from build123d import *

# Parameters (mm, degrees)
F0_W     = 1.2
F0_H     = 7
F1_DEPTH = 1.3
F2_DEPTH = 4.9
F3_DEPTH = 4


with BuildPart() as f1:
    # F0 (on Top) → F1 (new body)
    with BuildSketch(Plane.XY):
        with BuildLine():
            Line((9.05, 3.5), (6.914658, 3.5))
            ThreePointArc((6.914658, 3.5), (-4.806972, 6.079105), (-5, -5.92136))
            ThreePointArc((-5, -5.92136), (0, -7.75), (5, -5.92136))
            ThreePointArc((5, -5.92136), (6.079105, -4.806972), (6.914658, -3.5))
            Line((6.914658, -3.5), (9.05, -3.5))
            Line((9.05, -3.5), (9.05, 3.5))
        make_face()
        with BuildLine():
            ThreePointArc((-5, -5.92136), (-4.806972, 6.079105), (6.914658, 3.5))
            Line((6.914658, 3.5), (9.05, 3.5))
            Line((9.05, 3.5), (10.25, 3.5))
            Line((10.25, 3.5), (10.25, 4.5))
            Line((10.25, 4.5), (7.966963, 4.5))
            ThreePointArc((7.966963, 4.5), (-6.259851, 6.673588), (-5, -7.663061))
            Line((-5, -7.663061), (-5, -5.92136))
        make_face()
        with BuildLine():
            ThreePointArc((5, -5.92136), (0, -7.75), (-5, -5.92136))
            Line((-5, -5.92136), (-5, -7.663061))
            ThreePointArc((-5, -7.663061), (0, -9.15), (5, -7.663061))
            Line((5, -7.663061), (5, -5.92136))
        make_face()
        with Locations((9.65, 0)):
            Rectangle(F0_W, F0_H)
        with BuildLine():
            ThreePointArc((6.914658, -3.5), (6.079105, -4.806972), (5, -5.92136))
            Line((5, -5.92136), (5, -7.663061))
            ThreePointArc((5, -7.663061), (6.673588, -6.259851), (7.966963, -4.5))
            Line((7.966963, -4.5), (10.25, -4.5))
            Line((10.25, -4.5), (10.25, -3.5))
            Line((10.25, -3.5), (9.05, -3.5))
            Line((9.05, -3.5), (6.914658, -3.5))
        make_face()
    extrude(amount=F1_DEPTH)

    # F0 (on Top) → F2 (join)
    with BuildSketch(Plane.XY):
        with BuildLine():
            ThreePointArc((-5, -5.92136), (-4.806972, 6.079105), (6.914658, 3.5))
            Line((6.914658, 3.5), (9.05, 3.5))
            Line((9.05, 3.5), (10.25, 3.5))
            Line((10.25, 3.5), (10.25, 4.5))
            Line((10.25, 4.5), (7.966963, 4.5))
            ThreePointArc((7.966963, 4.5), (-6.259851, 6.673588), (-5, -7.663061))
            Line((-5, -7.663061), (-5, -5.92136))
        make_face()
        with BuildLine():
            ThreePointArc((6.914658, -3.5), (6.079105, -4.806972), (5, -5.92136))
            Line((5, -5.92136), (5, -7.663061))
            ThreePointArc((5, -7.663061), (6.673588, -6.259851), (7.966963, -4.5))
            Line((7.966963, -4.5), (10.25, -4.5))
            Line((10.25, -4.5), (10.25, -3.5))
            Line((10.25, -3.5), (9.05, -3.5))
            Line((9.05, -3.5), (6.914658, -3.5))
        make_face()
    extrude(amount=F2_DEPTH)

    # F0 (on Top) → F3 (join)
    with BuildSketch(Plane.XY):
        with Locations((9.65, 0)):
            Rectangle(F0_W, F0_H)
    extrude(amount=F3_DEPTH)


solid = f1.part
Model file for the job. Use its own axes, mm. A direction names the side the tool comes from. Give positions to 0.01 mm unless a question says otherwise; leave off trailing zeros. Write each loop counter-clockwise with the first axis right and the second up, starting at its lowest first coordinate (ties: lowest second). Pieces come first, ordered by that corner, then holes. Notation, with made-up numbers: (1.5, 62) -> (45.5, 62) arc R27 cw to (45.5, 99) -> close; hole circle Ø10 at (-20.75, -19.75). An arc over 180 degrees is marked (long way). Write item = value, one per line.
(1) Slice it at B-B, the plane z = 2.4. Give the cut face in (x, y).
Determined:
outline = (-5, -7.66) -> (-5, -5.92) arc R7.75 cw (long way) to (6.91, 3.5) -> (9.05, 3.5) -> (9.05, -3.5) -> (6.91, -3.5) arc R7.75 cw to (5, -5.92) -> (5, -7.66) arc R9.15 ccw to (7.97, -4.5) -> (10.25, -4.5) -> (10.25, 4.5) -> (7.97, 4.5) arc R9.15 ccw (long way) to start
(2) Slice it at C-C, the plane y = 0. Give the cut face in (x, z).
Determined:
outline = (-9.15, 0) -> (10.25, 0) -> (10.25, 4) -> (9.05, 4) -> (9.05, 1.3) -> (-7.75, 1.3) -> (-7.75, 4.9) -> (-9.15, 4.9) -> close
(3) Slice it at A-A, the plane x = 8.25. Give the cut face in (y, z), then the cut area to 3 significant figures.
Determined:
outline = (-4.5, 0) -> (4.5, 0) -> (4.5, 4.9) -> (3.5, 4.9) -> (3.5, 1.3) -> (-3.5, 1.3) -> (-3.5, 4.9) -> (-4.5, 4.9) -> close
area = 18.9 mm2
(4) Tool access for faces 1 (the face through (9, 4.5, 2)), 2 (the face through (6.09, -4.79, 3.07)), 3 (the face through (-5, -7, 3)): list every direction of +Z, -Z, +X, -X, +Y, -Y with a clear straight run to the whole face (end or side of a thin tool).
Determined:
face_1 = +Z, -Z, +X, +Y
face_2 = +Z
face_3 = +Z, -Y
(5) Flat gauge pins, fed straight in: P1, Ø5, axis at x = 1, y = 2, coming from the +Z side; P2, Ø0.7, axis at x = 9, z = 3, coming from the +Y side; P3, Ø1.7, axis at x = 9, z = 4, coming from the -Y side. Where does each tip first touch, or does it go through?
Determined:
P1 = 1.3
P2 = 4.5
P3 = -4.5
(6) Mould opens along Y. For faces 4 (the face through (10, 0, 4)), 5 (the face through (9.05, 0, 3)), 6 (the face through (9, -4.5, 2)), 7 (the face through (10.25, 0, 2)) say: released by +Y, released by -Y, zero draft, split by the parting line, or undercut.
Determined:
face_4 = undercut
face_5 = undercut
face_6 = released by -Y
face_7 = zero draft
(7) Probe line 1 along X through (y, z) = (0, 3.85); line 2 along Y through (x, z) = (0, 4.1); line 3 along Z through (x, y) = (-7, -0.25). List the from-to ranges inside material, lowest first.
Determined:
line_1 = -9.15 to -7.75, 9.05 to 10.25
line_2 = 7.75 to 9.15
line_3 = 0 to 1.3
(8) Slice it at D-D, the plane x = 0. Give the cut face in (y, z), then the cut area to 3 significant figures.
Determined:
outline = (-9.15, 0) -> (9.15, 0) -> (9.15, 4.9) -> (7.75, 4.9) -> (7.75, 1.3) -> (-9.15, 1.3) -> close
area = 28.8 mm2
